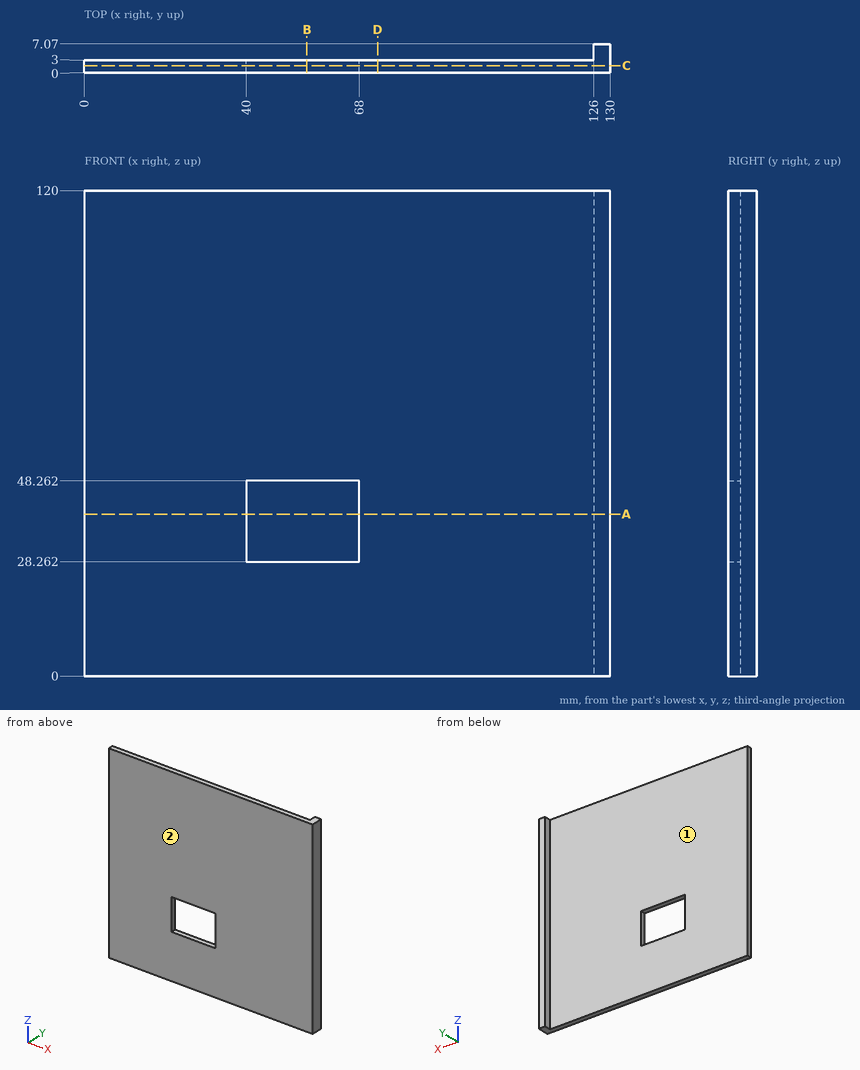
Study the drawing (mm; zero at the part's minimum x, y, z) and answer. A direction names the side the tool comes from. Coordinates: 2 decimals unless noted, no trailing zeros. Loops run counter-clockwise (first coordinate to the right, second up) from the corner with the lowest first, then second, coordinate; pieces in that order, holes last. Notation, with made-up numbers: M 78.25,17 L 118.25,17 A30 ccw 118.25,50 Z; hole C 27.5,60.25 d9. An arc over 180 degrees is marked long. Answer as a JSON object with one key per item and string values. Group by question number.
Item 1: Which of the six approach directions +Z, -Z, +X, -X, +Y, -Y give full straight-line access (tool end or side, diameter ignored) to the marked faces 1 and 2?
Item 2: Consider L1, parallel to Z at x = 43, y = 0.5; L2, parallel to Y at x = 92, z = 25.5; L3, parallel to X at y = 6, z = 8. Determine where each line is inside the solid, lowest interval first.
Item 3: Each of these flat-tipped pins is pushed along its axis until it touches: P1, Ø8, axis at x = 109.5, z = 77.5, coming from the +Y side; P2, Ø1, axis at y = 5, z = 30, coming from the -X side. Where does it stop, or does it pass through?
Item 4: Section D-D (x = 72.5) is taken. Write down the section's boundary in (y, z), and give its area (3 significant figures).
Item 5: Section B-B (x = 55) is taken. Write down the section's boundary in (y, z).
Item 6: Section C-C (y = 1.75) is taken. Write down the section's boundary in (x, z).
Item 7: Section A-A (z = 40) is taken. Write down the section's boundary in (x, y).
Solved:
{
 "1": {"face 1": "+Z, -Z, -X, +Y", "face 2": "+Z, -Z, +X, -X, -Y"},
 "2": {"L1": "z = 0 to 28.26, 48.26 to 120", "L2": "y = 0 to 3", "L3": "x = 126 to 130"},
 "3": {"P1": "stops at y = 3", "P2": "stops at x = 126"},
 "4": {"outline": "M 0,0 L 3,0 L 3,120 L 0,120 Z", "area": "360 mm2"},
 "5": {"outline": "M 0,0 L 3,0 L 3,28.26 L 0,28.26 Z; M 0,48.26 L 3,48.26 L 3,120 L 0,120 Z"},
 "6": {"outline": "M 0,0 L 130,0 L 130,120 L 0,120 Z; hole M 40,28.26 L 68,28.26 L 68,48.26 L 40,48.26 Z"},
 "7": {"outline": "M 0,0 L 40,0 L 40,3 L 0,3 Z; M 68,0 L 130,0 L 130,7.07 L 126,7.07 L 126,3 L 68,3 Z"}
}
